Check sheet for the drawn part. Datum: minimum x, y, z corner. Units: mm. A direction names the side the tool comes from. Give positions to 0.01 mm unless a question says otherwise; leave off trailing zeros. Order: outer loops, then holes, each group sorted by start corner. A loop starts at its lowest first (then second) coordinate and runs counter-clockwise, first axis right, second up. Notation, with made-up numbers: (32, 41.25) - (85, 41.25) arc R7 ccw to (85, 50.25) - close; hole circle Ø6 at (56.5, -16.75). An arc over 180 degrees is marked (long way). Answer as a JSON object with one key per item and string values. Group by question number.
(1) Access from +Z, -Z, +X, -X, +Y, -Y to the whole of each face (thin tool, end or side, straight path). Record for the marked faces 1, 2, 3, 4 and 5.
(2) Section check A-A (z = 56). Record the boundary of the cut face in (x, y), then the cut area to 3 significant figures.
(3) Section check C-C (z = 31.75). Record the boundary of the cut face in (x, y), then the cut area to 3 significant figures.
(4) Depth check by flat-ended pin: pin 1 Ø3 at (x, z) = (90, 29) entering from -Y; pin 2 Ø1 at (x, y) = (39, 1.5) entering from +Z; pin 3 Ø2 at (x, y) = (83.5, 8) entering from +Z; pin 4 Ø1 at (x, y) = (23, 4) entering from -Z. Enter the tip coordinate at first touch or a pass-through.
(5) Section check B-B (y = 7). Count the separate pieces of the cut face and the enclosed holes in it, then the cut area to 3 significant figures.
(6) Section check D-D (x = 104.5). Record the boundary of the cut face in (y, z), then the cut area to 3 significant figures.
(7) Thickness scan on line 1 (Z direction, x = 95.25, y = 7) (1 decimal); line 2 (X direction, y = 2.5, z = 8); line 3 (X direction, y = 8.5, z = 53). Record the ranges inside material, lowest first.
(8) Mould release check, pull along Z, two halves, no side actions. Record for the marked faces 6, 7 and 8: +Z half, -Z half, draft (parallel to the pull), parting line (faces both ways), or undercut.
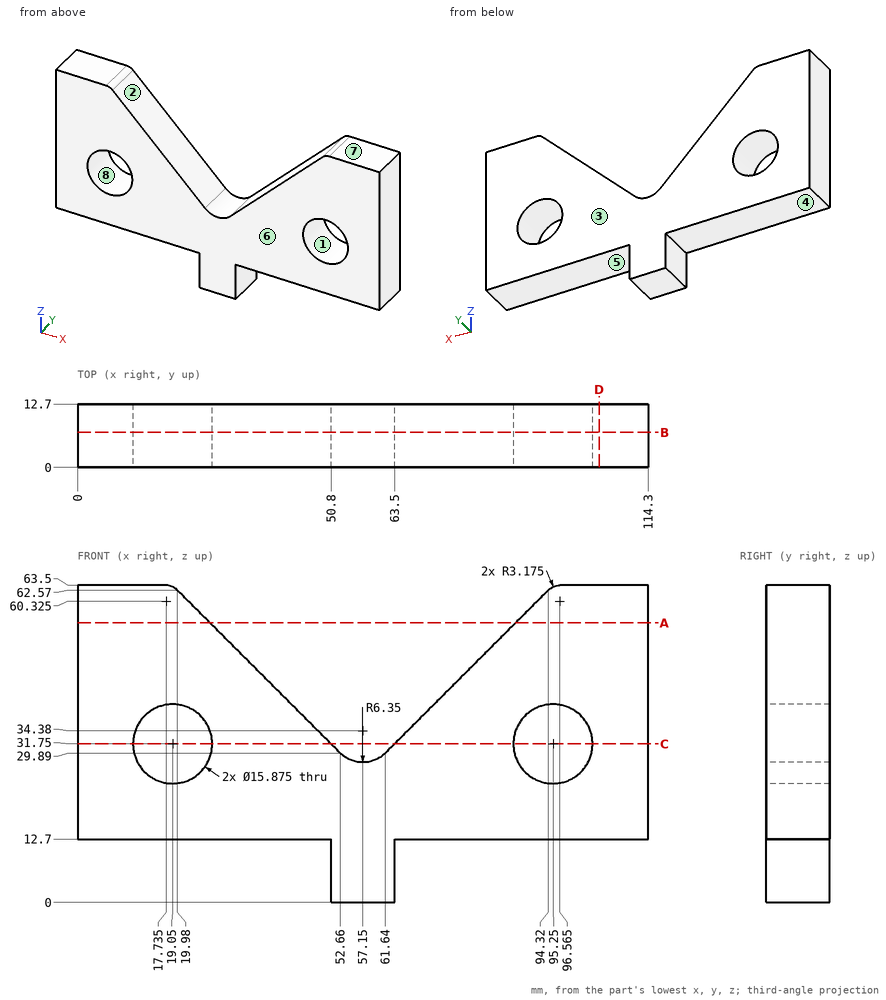
Solutions:
{
 "1": {"face 1": "+Y, -Y", "face 2": "+Z, +Y, -Y", "face 3": "+Z, -Z, +X, -X, +Y", "face 4": "-Z, -X, +Y, -Y", "face 5": "-Z, +X, +Y, -Y"},
 "2": {"outline": "(0, 0) - (26.55, 0) - (26.55, 12.7) - (0, 12.7) - close; (87.75, 0) - (114.3, 0) - (114.3, 12.7) - (87.75, 12.7) - close", "area": "674 mm2"},
 "3": {"outline": "(0, 0) - (11.11, 0) - (11.11, 12.7) - (0, 12.7) - close; (26.99, 0) - (50.8, 0) - (50.8, 12.7) - (26.99, 12.7) - close; (63.5, 0) - (87.31, 0) - (87.31, 12.7) - (63.5, 12.7) - close; (103.19, 0) - (114.3, 0) - (114.3, 12.7) - (103.19, 12.7) - close", "area": "887 mm2"},
 "4": {"pin 1": "passes through", "pin 2": "stops at z = 44.05", "pin 3": "stops at z = 52.75", "pin 4": "stops at z = 12.7"},
 "5": {"separate pieces": "1", "enclosed holes": "2", "area": "4,130 mm2"},
 "6": {"outline": "(0, 12.7) - (12.7, 12.7) - (12.7, 63.5) - (0, 63.5) - close", "area": "645 mm2"},
 "7": {"line 1": "z = 12.7 to 23.8, 39.7 to 63.2", "line 2": "x = 50.8 to 63.5", "line 3": "x = 0 to 29.55, 84.75 to 114.3"},
 "8": {"face 6": "draft", "face 7": "+Z half", "face 8": "undercut"}
}
